Part model, mm, in its own coordinate system. A direction names the side the tool comes from. Coordinates: 2 decimals unless noted, no trailing zeros. Order: outer loops, then holes, each group sorted by start corner. A loop starts at its lowest first (then second) coordinate and runs counter-clockwise, first axis right, second up.
1) Cut at C-C (z = 1.25). Give the number of separate pieces and of enclosed holes in the cut face, and give its area (3 significant figures).
2) Pin check, flat tips, straight feed: pin 1 Ø1.8 at (x, z) = (87.5, 3) entering from +Y; pin 2 Ø1.7 at (y, z) = (2, 2.5) entering from -X; pin 3 Ø0.8 at (x, z) = (-1, 2) entering from -Y. Stop position of each tip, or through.
3) Wall check: L1, parallel to Y at x = 25.5, z = 7; L2, parallel to X at y = 40.5, z = 16.75; L3, parallel to Z at x = 52.5, y = 14. Give the ranges that are in metal, low to high.
4) Mould opens along Y. For faces 4 (the flat face through (40, -2.8, 9)), 5 (the flat face through (40, 57.41, 9)), 6 (the flat face through (-2, 37.85, 12)) say: +Y half, -Y half, draft (parallel to the pull), parting line (faces both ways), or undercut.
5) Tool access for faces 1 (the cylindrical face through (84.74, 1.86, 8.97)), 2 (the flat face through (-2, 44, 4)), 3 (the cylindrical face through (14.545, 5.924, 1.972)): list every direction of +Z, -Z, +X, -X, +Y, -Y with a clear straight run to the whole face (end or side of a thin tool).
6) Cut at A-A (z = 15.25). List the corners of the cut face in (x, y).
7) Cut at B-B (x = 59.5). List the corners of the cut face in (y, z).
```python
from build123d import *

# Parameters (mm, degrees)
SKETCH5_R                    = 1.25
BOTTOM_FRAME_DEPTH           = 4
PCB_DEPTH                    = 1.6
SKETCH7_W                    = 2.5
SKETCH7_H                    = 7.1
UPPER_FRAME_DEPTH            = 15
BOTTOM_DEPTH                 = 3
SKETCH9_W                    = 2.5
SKETCH9_H                    = 16.5
NETWORK_CONNECTOR_BOSS_DEPTH = 1.3
BOSS_EXTRUDE8_DEPTH          = 3.7
MINI_USB_REACH               = 93.96
SKETCH11_W                   = 3.9
SKETCH11_H                   = 7.7
CUT_EXTRUDE3_REACH           = 93.96
SKETCH12_W                   = 1.61
SKETCH12_H                   = 12


with BuildPart() as part:
    # Sketch5 → Bottom frame (new body)
    with BuildSketch(Plane.XY):
        with BuildLine():
            Line((73.66, 57.41), (6.35, 57.41))
            ThreePointArc((6.35, 57.41), (-0.120027048, 54.730027048), (-2.8, 48.26))
            Line((-2.8, 48.26), (-2.8, 6.35))
            ThreePointArc((-2.8, 6.35), (-0.120027048, -0.120027048), (6.35, -2.8))
            Line((6.35, -2.8), (73.66, -2.8))
            ThreePointArc((73.66, -2.8), (84.620155108, 1.739844892), (89.16, 12.7))
            Line((89.16, 12.7), (89.16, 41.91))
            ThreePointArc((89.16, 41.91), (84.620155108, 52.870155108), (73.66, 57.41))
        make_face()
        with Locations((14.605, 51.435)):
            Circle(SKETCH5_R, mode=Mode.SUBTRACT)
        with Locations((80.645, 48.26)):
            Circle(SKETCH5_R, mode=Mode.SUBTRACT)
        with Locations((80.645, 6.35)):
            Circle(SKETCH5_R, mode=Mode.SUBTRACT)
        with Locations((14.605, 3.175)):
            Circle(SKETCH5_R, mode=Mode.SUBTRACT)
        with BuildLine():
            Line((73.66, 54.91), (17.355, 54.91))
            Line((17.355, 54.91), (17.355, 51.435))
            ThreePointArc((17.355, 51.435), (14.605, 48.685), (11.855, 51.435))
            Line((11.855, 51.435), (11.855, 54.91))
            Line((11.855, 54.91), (6.35, 54.91))
            ThreePointArc((6.35, 54.91), (1.647739905, 52.962260095), (-0.3, 48.26))
            Line((-0.3, 48.26), (-0.3, 6.35))
            ThreePointArc((-0.3, 6.35), (1.647739905, 1.647739905), (6.35, -0.3))
            Line((6.35, -0.3), (11.855, -0.3))
            Line((11.855, -0.3), (11.855, 3.175))
            ThreePointArc((11.855, 3.175), (14.605, 5.925), (17.355, 3.175))
            Line((17.355, 3.175), (17.355, -0.3))
            Line((17.355, -0.3), (73.66, -0.3))
            ThreePointArc((73.66, -0.3), (75.806982263, -0.121484593), (77.895, 0.409158898))
            Line((77.895, 0.409158898), (77.895, 6.35))
            ThreePointArc((77.895, 6.35), (78.700456352, 8.294543648), (80.645, 9.1))
            Line((80.645, 9.1), (86.151597176, 9.1))
            ThreePointArc((86.151597176, 9.1), (86.532271814, 10.882139071), (86.66, 12.7))
            Line((86.66, 12.7), (86.66, 41.91))
            ThreePointArc((86.66, 41.91), (86.532271814, 43.727860929), (86.151597176, 45.51))
            Line((86.151597176, 45.51), (80.645, 45.51))
            ThreePointArc((80.645, 45.51), (78.700456352, 46.315456352), (77.895, 48.26))
            Line((77.895, 48.26), (77.895, 54.200841102))
            ThreePointArc((77.895, 54.200841102), (75.806982263, 54.731484593), (73.66, 54.91))
        make_face(mode=Mode.SUBTRACT)
    extrude(amount=BOTTOM_FRAME_DEPTH)

    # Sketch6 → PCB (add)
    with BuildSketch(Plane.XY.offset(4)):
        with BuildLine():
            Line((73.66, 57.41), (6.35, 57.41))
            ThreePointArc((6.35, 57.41), (-0.120027048, 54.730027048), (-2.8, 48.26))
            Line((-2.8, 48.26), (-2.8, 6.35))
            ThreePointArc((-2.8, 6.35), (-0.120027048, -0.120027048), (6.35, -2.8))
            Line((6.35, -2.8), (73.66, -2.8))
            ThreePointArc((73.66, -2.8), (84.620155108, 1.739844892), (89.16, 12.7))
            Line((89.16, 12.7), (89.16, 41.91))
            ThreePointArc((89.16, 41.91), (84.620155108, 52.870155108), (73.66, 57.41))
        make_face()
        with BuildLine():
            Line((-0.3, 48.26), (-0.3, 6.35))
            ThreePointArc((-0.3, 6.35), (1.647739905, 1.647739905), (6.35, -0.3))
            Line((6.35, -0.3), (73.66, -0.3))
            ThreePointArc((73.66, -0.3), (82.852388155, 3.507611845), (86.66, 12.7))
            Line((86.66, 12.7), (86.66, 41.91))
            ThreePointArc((86.66, 41.91), (82.852388155, 51.102388155), (73.66, 54.91))
            Line((73.66, 54.91), (6.35, 54.91))
            ThreePointArc((6.35, 54.91), (1.647739905, 52.962260095), (-0.3, 48.26))
        make_face(mode=Mode.SUBTRACT)
    extrude(amount=PCB_DEPTH)

    # Sketch7 → upper frame (add)
    with BuildSketch(Plane.XY.offset(5.6)):
        with BuildLine():
            Line((6.35, 54.91), (73.66, 54.91))
            ThreePointArc((73.66, 54.91), (82.852388155, 51.102388155), (86.66, 41.91))
            Line((86.66, 41.91), (86.66, 12.7))
            ThreePointArc((86.66, 12.7), (82.852388155, 3.507611845), (73.66, -0.3))
            Line((73.66, -0.3), (6.35, -0.3))
            ThreePointArc((6.35, -0.3), (2.252287223, 1.112514916), (-0.104649487, 4.75))
            Line((-0.104649487, 4.75), (-2.659023254, 4.75))
            ThreePointArc((-2.659023254, 4.75), (0.472819554, -0.662934479), (6.35, -2.8))
            Line((6.35, -2.8), (73.66, -2.8))
            ThreePointArc((73.66, -2.8), (84.620155108, 1.739844892), (89.16, 12.7))
            Line((89.16, 12.7), (89.16, 41.91))
            ThreePointArc((89.16, 41.91), (84.620155108, 52.870155108), (73.66, 57.41))
            Line((73.66, 57.41), (6.35, 57.41))
            ThreePointArc((6.35, 57.41), (-0.120027048, 54.730027048), (-2.8, 48.26))
            Line((-2.8, 48.26), (-2.8, 37.85))
            Line((-2.8, 37.85), (-0.3, 37.85))
            Line((-0.3, 37.85), (-0.3, 48.26))
            ThreePointArc((-0.3, 48.26), (1.647739905, 52.962260095), (6.35, 54.91))
        make_face()
        with Locations((-1.55, 17.8)):
            Rectangle(SKETCH7_W, SKETCH7_H)
    extrude(amount=UPPER_FRAME_DEPTH)

    # Sketch8 → bottom (add)
    with BuildSketch(Plane(origin=(0, 0, 0), x_dir=(-1, 0, 0), z_dir=(0, 0, -1))):
        with BuildLine():
            Line((-89.16, 41.91), (-89.16, 12.7))
            ThreePointArc((-89.16, 12.7), (-84.620155108, 1.739844892), (-73.66, -2.8))
            Line((-73.66, -2.8), (-6.35, -2.8))
            ThreePointArc((-6.35, -2.8), (0.120027048, -0.120027048), (2.8, 6.35))
            Line((2.8, 6.35), (2.8, 48.26))
            ThreePointArc((2.8, 48.26), (0.120027048, 54.730027048), (-6.35, 57.41))
            Line((-6.35, 57.41), (-73.66, 57.41))
            ThreePointArc((-73.66, 57.41), (-84.620155108, 52.870155108), (-89.16, 41.91))
        make_face()
    extrude(amount=BOTTOM_DEPTH)

    # Sketch9 → network connector boss (add)
    with BuildSketch(Plane.XY.offset(20.6)):
        with Locations((-1.55, 29.6)):
            Rectangle(SKETCH9_W, SKETCH9_H)
    extrude(amount=-NETWORK_CONNECTOR_BOSS_DEPTH)

    # Sketch10 → Boss-Extrude8 (add)
    with BuildSketch(Plane.XY.offset(20.6)):
        with BuildLine():
            Line((-0.3, 14.25), (-2.8, 14.25))
            Line((-2.8, 14.25), (-2.8, 6.35))
            ThreePointArc((-2.8, 6.35), (-2.764687674, 5.546900622), (-2.659023254, 4.75))
            Line((-2.659023254, 4.75), (-0.104649487, 4.75))
            ThreePointArc((-0.104649487, 4.75), (-0.250981711, 5.544059273), (-0.3, 6.35))
            Line((-0.3, 6.35), (-0.3, 14.25))
        make_face()
    extrude(amount=-BOSS_EXTRUDE8_DEPTH)

    # Sketch11 → mini-USB (cut, up to next)
    with BuildSketch(Plane.ZY.offset(2.8), mode=Mode.PRIVATE) as mini_usb_sk1:
        with Locations((2.05, 44.21)):
            Rectangle(SKETCH11_W, SKETCH11_H)
    mini_usb_tool1 = extrude(mini_usb_sk1.sketch, amount=-MINI_USB_REACH, mode=Mode.PRIVATE) & part.part
    add(mini_usb_tool1.solids().sort_by_distance((-2.8, 44.21, 2.05))[0], mode=Mode.SUBTRACT)

    # Sketch12 → Cut-Extrude3 (cut, up to next)
    with BuildSketch(Plane(origin=(89.16, 0, 0), x_dir=(0, 0, -1), z_dir=(1, 0, 0)), mode=Mode.PRIVATE) as cut_extrude3_sk1:
        with Locations((-3.195, 37.11)):
            Rectangle(SKETCH12_W, SKETCH12_H)
    cut_extrude3_tool1 = extrude(cut_extrude3_sk1.sketch, amount=-CUT_EXTRUDE3_REACH, mode=Mode.PRIVATE) & part.part
    add(cut_extrude3_tool1.solids().sort_by_distance((89.16, 37.11, 3.195))[0], mode=Mode.SUBTRACT)


solid = part.part
```
Geometry check:
1. separate pieces: 1
1. enclosed holes: 4
1. area: 804 mm2
2. pin 1: stops at y = 50.44
2. pin 2: stops at x = -2.1
2. pin 3: stops at y = 0.4
3. L1: y = -2.8 to -0.3, 54.91 to 57.41
3. L2: x = -2.8 to -0.3, 86.66 to 89.16
3. L3: z = -3 to 0
4. face 4: -Y half
4. face 5: +Y half
4. face 6: undercut
5. face 1: +Z, -Z, +X, -Y
5. face 2: -X
5. face 3: +Z
6. outline: (-2.8, 14.25) - (-0.3, 14.25) - (-0.3, 21.35) - (-2.8, 21.35) - close; (-2.8, 37.85) - (-0.3, 37.85) - (-0.3, 48.26) arc R6.65 cw to (6.35, 54.91) - (73.66, 54.91) arc R13 cw to (86.66, 41.91) - (86.66, 12.7) arc R13 cw to (73.66, -0.3) - (6.35, -0.3) arc R6.65 cw to (-0.1, 4.75) - (-2.66, 4.75) arc R9.15 ccw to (6.35, -2.8) - (73.66, -2.8) arc R15.5 ccw to (89.16, 12.7) - (89.16, 41.91) arc R15.5 ccw to (73.66, 57.41) - (6.35, 57.41) arc R9.15 ccw to (-2.8, 48.26) - close
7. outline: (-2.8, -3) - (57.41, -3) - (57.41, 20.6) - (54.91, 20.6) - (54.91, 0) - (-0.3, 0) - (-0.3, 20.6) - (-2.8, 20.6) - close
